Check sheet for the modelled part. Datum: model origin and axes. Units: mm. Round coordinates to 2 decimals unless told otherwise and drop trailing zeros. Order: outer loops, then holes, each group sorted by start corner. A loop starts at its lowest first (then second) coordinate and runs counter-clockwise, first axis right, second up.
(1) Sectioned sample at B-B, the plane y = 0.85. Enter the section's corners in (x, z) (3 decimals), and give its area (3 significant figures).
(2) Thickness scan on probe 1 along Z at (x, y) = (27.3, 0.65); probe 2 along Z at (x, y) = (26, 0.5); probe 3 along X at (y, z) = (0.65, 7.75) (3 decimals). Record the ranges inside material, lowest first.
(3) Sectioned sample at A-A, the plane x = 27.3. Enter the section's corners in (y, z).
(4) Sectioned sample at C-C, the plane x = 16. Enter the section's corners in (y, z), and give its area (3 significant figures).
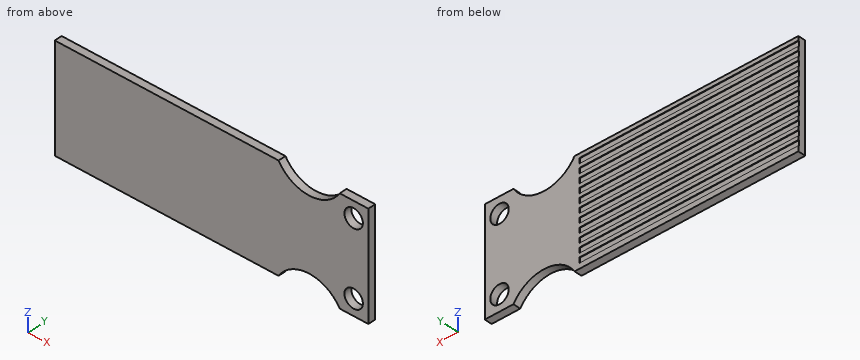
```python
from build123d import *

# Parameters (mm, degrees)
BOSS_EXTRUDE1_DEPTH = 1.45
SKETCH2_R           = 1.775
CUT_EXTRUDE1_DEPTH  = 2.45
SKETCH3_W           = 42.044311255
SKETCH3_H           = 1
CUT_EXTRUDE2_DEPTH  = 0.1


with BuildPart() as part:
    # Sketch1 → Boss-Extrude1 (new body)
    with BuildSketch(Plane(origin=(0, 0, 0), x_dir=(1, 0, 0), z_dir=(0, 1, 0))):
        with BuildLine():
            Line((-30.125, -10.15), (12.875, -10.15))
            ThreePointArc((12.875, -10.15), (18.75, -6.862513487), (24.625, -10.15))
            Line((24.625, -10.15), (30.125, -10.15))
            Line((30.125, -10.15), (30.125, 10.15))
            Line((30.125, 10.15), (24.625, 10.15))
            ThreePointArc((24.625, 10.15), (18.75, 6.862513487), (12.875, 10.15))
            Line((12.875, 10.15), (-30.125, 10.15))
            Line((-30.125, 10.15), (-30.125, -10.15))
        make_face()
    extrude(amount=BOSS_EXTRUDE1_DEPTH)

    # Sketch2 → Cut-Extrude1 (cut, through all)
    with BuildSketch(Plane(origin=(0, 1.45, 0), x_dir=(1, 0, 0), z_dir=(0, 1, 0))):
        with Locations((27.3, 7.075)):
            Circle(SKETCH2_R)
        with Locations((27.3, -7.075)):
            Circle(SKETCH2_R)
    extrude(amount=-CUT_EXTRUDE1_DEPTH, mode=Mode.SUBTRACT)

    # Sketch3 → Cut-Extrude2 (cut)
    with BuildSketch(Plane(origin=(0, 1.45, 0), x_dir=(1, 0, 0), z_dir=(0, 1, 0))):
        with Locations((-9.102844373, 8.65)):
            Rectangle(SKETCH3_W, SKETCH3_H)
        with Locations((-9.102844373, 6.9)):
            Rectangle(SKETCH3_W, SKETCH3_H)
        with Locations((-9.102844373, 5.15)):
            Rectangle(SKETCH3_W, SKETCH3_H)
        with Locations((-9.102844373, 3.4)):
            Rectangle(SKETCH3_W, SKETCH3_H)
        with Locations((-9.102844373, 1.65)):
            Rectangle(SKETCH3_W, SKETCH3_H)
        with Locations((-9.102844373, -0.1)):
            Rectangle(SKETCH3_W, SKETCH3_H)
        with Locations((-9.102844373, -1.85)):
            Rectangle(SKETCH3_W, SKETCH3_H)
        with Locations((-9.102844373, -3.6)):
            Rectangle(SKETCH3_W, SKETCH3_H)
        with Locations((-9.102844373, -5.35)):
            Rectangle(SKETCH3_W, SKETCH3_H)
        with Locations((-9.102844373, -7.1)):
            Rectangle(SKETCH3_W, SKETCH3_H)
        with Locations((-9.102844373, -8.85)):
            Rectangle(SKETCH3_W, SKETCH3_H)
    extrude(amount=-CUT_EXTRUDE2_DEPTH, mode=Mode.SUBTRACT)


solid = part.part
```
Derived:
1. outline: (-30.125, -10.15) - (12.875, -10.15) arc R6.893 cw to (24.625, -10.15) - (30.125, -10.15) - (30.125, 10.15) - (24.625, 10.15) arc R6.893 cw to (12.875, 10.15) - (-30.125, 10.15) - close; hole circle Ø3.55 at (27.3, -7.075); hole circle Ø3.55 at (27.3, 7.075)
1. area: 1,150 mm2
2. probe 1: z = -10.15 to -8.85, -5.3 to 5.3, 8.85 to 10.15
2. probe 2: z = -10.15 to -8.28, -5.87 to 5.87, 8.28 to 10.15
2. probe 3: x = -30.125 to 15.367, 22.133 to 25.658, 28.942 to 30.125
3. outline: (0, -10.15) - (1.45, -10.15) - (1.45, -8.85) - (0, -8.85) - close; (0, -5.3) - (1.45, -5.3) - (1.45, 5.3) - (0, 5.3) - close; (0, 8.85) - (1.45, 8.85) - (1.45, 10.15) - (0, 10.15) - close
4. outline: (0, -7.43) - (1.45, -7.43) - (1.45, 7.43) - (0, 7.43) - close
4. area: 21.6 mm2
